Source: three-view drawing plus pictorial views. Frame: mm from the lowest corner of the part. Give positions to 0.01 mm unless a question says otherwise; leave off trailing zeros. Order: outer loops, then holes, each group sorted by start corner. A loop starts at its lowest first (then second) coordinate and runs counter-clockwise, first axis right, second up.
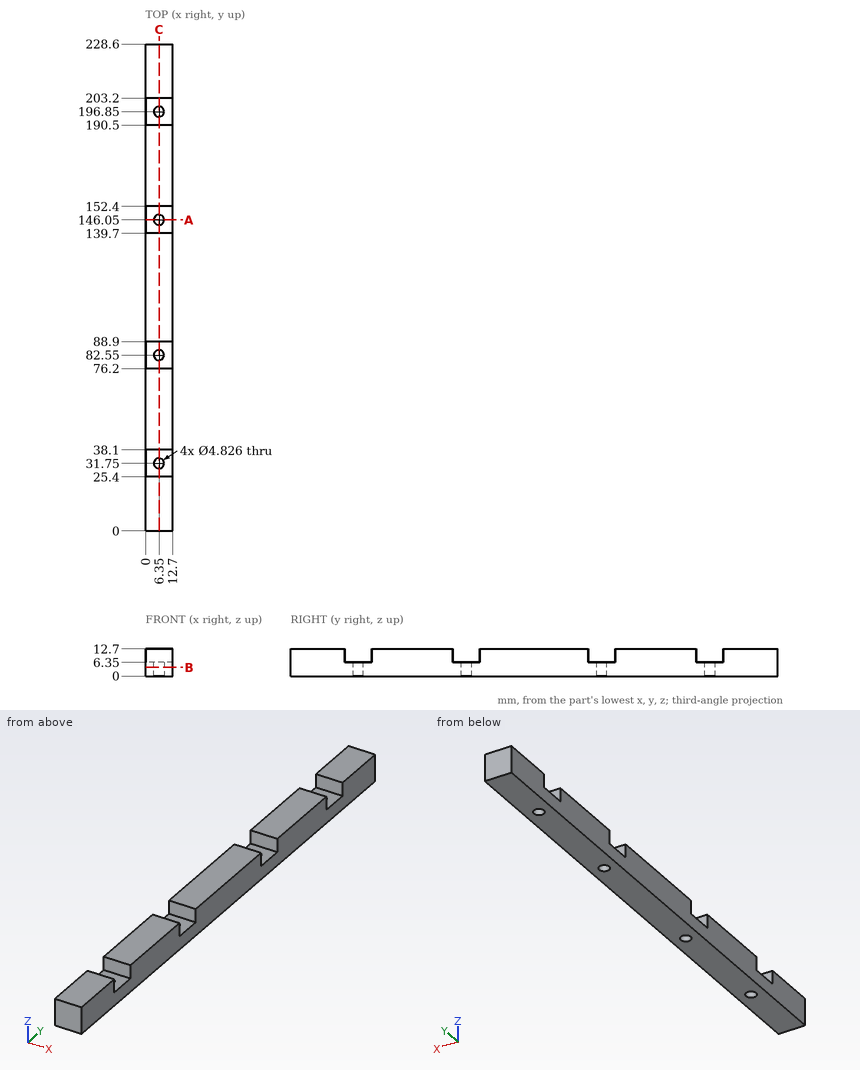
(1) Section C-C, the plane x = 6.35. Count the separate pieces of the cut face and the enclosed holes in it, plus the area to 3 significant figures.
(2) Section A-A, the plane y = 146.05. Return loops of the section in (x, z).
(3) Line query: line 1 along Y through (x, z) = (6.35, 1.5); line 2 along Y through (x, z) = (6, 10); line 3 along X through (y, z) = (146.05, 2). Output: solid intervals per line, ascending.
(4) Section B-B, the plane z = 4. Return loops of the section in (x, y), plus the area to 3 significant figures.
(5) Pin query (flat end, axial travel): pin 1 Ø1 at (y, z) = (151.5, 10) entering from -X; pin 2 Ø4 at (x, y) = (9.5, 147) entering from +Z; pin 3 Ø4 at (x, y) = (5.5, 198.5) entering from +Z. Return the tip coordinate at first contact, or that it passes through.
Checks:
1. separate pieces: 5
1. enclosed holes: 0
1. area: 2,460 mm2
2. outline: (0, 0) - (3.94, 0) - (3.94, 6.35) - (0, 6.35) - close; (8.76, 0) - (12.7, 0) - (12.7, 6.35) - (8.76, 6.35) - close
3. line 1: y = 0 to 29.34, 34.16 to 80.14, 84.96 to 143.64, 148.46 to 194.44, 199.26 to 228.6
3. line 2: y = 0 to 25.4, 38.1 to 76.2, 88.9 to 139.7, 152.4 to 190.5, 203.2 to 228.6
3. line 3: x = 0 to 3.94, 8.76 to 12.7
4. outline: (0, 0) - (12.7, 0) - (12.7, 228.6) - (0, 228.6) - close; hole circle Ø4.83 at (6.35, 31.75); hole circle Ø4.83 at (6.35, 82.55); hole circle Ø4.83 at (6.35, 146.05); hole circle Ø4.83 at (6.35, 196.85)
4. area: 2,830 mm2
5. pin 1: passes through
5. pin 2: stops at z = 6.35
5. pin 3: stops at z = 6.35
